from build123d import *

# Parameters (mm, degrees)
F0_W     = 18.4755190939
F0_H     = 19.05
F1_DEPTH = 12.7
F2_DEPTH = 76.2
F4_DEPTH = 12.7
F3_W     = 19.05
F3_H     = 19.05
F5_DEPTH = 25.4


# Not quite as in the source:
# - a feature names something its author has since deleted; it is built from what else it names


with BuildPart() as f1:
    # F0 (on Top) → F1 (new body)
    with BuildSketch(Plane.XY):
        with BuildLine():
            Line((34.1462217655, 9.525), (-48.9782591407, 9.525))
            ThreePointArc((-48.9782591407, 9.525), (-58.5032591407, 0), (-48.9782591407, -9.525))
            Line((-48.9782591407, -9.525), (34.1462217655, -9.525))
            Line((34.1462217655, -9.525), (34.1462217655, 9.525))
        make_face()
        with Locations((43.3839813124, 0)):
            Rectangle(F0_W, F0_H)
    extrude(amount=F1_DEPTH)

    # F0 (on Top) → F2 (join)
    with BuildSketch(Plane.XY):
        with Locations((43.3839813124, 0)):
            Rectangle(F0_W, F0_H)
    extrude(amount=F2_DEPTH)

    # F3 (on face) → F4 (join)
    with BuildSketch(Plane.XY.offset(76.2)):
        Polygon((52.6217408593, -9.525), (34.1462217655, -9.525), (34.1462217655, -219.075), (53.1962217655, -219.075), (53.1962217655, -9.525), align=None)
    extrude(amount=-F4_DEPTH)

    # F3 (on face) → F5 (join)
    with BuildSketch(Plane.XY.offset(76.2)):
        with Locations((43.6712217655, -228.6)):
            Rectangle(F3_W, F3_H)
    extrude(amount=-F5_DEPTH)


with BuildPart() as f6_1:
    # F6: copy of F1
    add(f1.part)


solid = f1.part
Read the model definition and answer for the solid it produces. Units are mm, in the model's axes. A direction names the side the tool comes from. Give positions to 0.01 mm unless a question says otherwise; leave off trailing zeros. Loops run counter-clockwise (first coordinate to the right, second up) from the corner with the lowest first, then second, coordinate; pieces in that order, holes last. Notation, with made-up numbers: (88.25, 9) - (128.25, 9) arc R25 cw to (128.25, 21) - close; hole circle Ø11 at (81, 41.25). An arc over 180 degrees is marked (long way). Answer as CSV lines item,"result". Start each with the question number.
1) Determine the mould class of faces 1 (the face through (44, -113, 76.2)), 2 (the face through (44, -219.075, 57)), 3 (the face through (25, 9.525, 12)) for opening direction Y: released by +Y, released by -Y, zero draft, split by the parting line, or undercut.
2) Each of these flat-tipped pins is pushed along its axis until it touches: pin 1 Ø0.6 at (x, z) = (53, 72) entering from +Y (3 decimals); pin 2 Ø15 at (y, z) = (1, 24.5) entering from +X; pin 3 Ø21 at (x, y) = (41, -80) entering from -Z. Where does it stop, or does it pass through?
3) Straight lines are drawn through the part: L1, parallel to Z at x = 43, y = -100; L2, parallel to X at y = -29.5, z = 64.5; L3, parallel to Y at x = 40, z = 12.5 (3 decimals). For each, find the intervals that lie inside material, in ascending order. Write a range as from..to.
4) Find section A-A (x = 38). Write down the section's boundary in (y, z) (3 decimals).
5) Find section D-D (x = 23). Write down the section's boundary in (y, z) (3 decimals), then the cut area to 3 significant figures.
6) Which of the six approach directions +Z, -Z, +X, -X, +Y, -Y give full straight-line access (tool end or side, diameter ignored) to faces 4 (the face through (24, -9.525, 10)), 5 (the face through (44, -228, 50.8)), 6 (the face through (-13, 0, 12.7))?
7) Find section C-C (y = 0). Write down the section's boundary in (x, z).
8) Find section B-B (z = 20). Write down the section's boundary in (x, y) (3 decimals).
Findings below:
1,face 1,"zero draft"
1,face 2,"undercut"
1,face 3,"released by +Y"
2,pin 1,"y = -9.525"
2,pin 2,"x = 52.62"
2,pin 3,"z = 63.5"
3,L1,"63.5..76.2"
3,L2,"34.15..53.2"
3,L3,"-9.525..9.525"
4,outline,"(-238.125, 50.8) - (-219.075, 50.8) - (-219.075, 63.5) - (-9.525, 63.5) - (-9.525, 0) - (9.525, 0) - (9.525, 76.2) - (-238.125, 76.2) - close"
5,outline,"(-9.525, 0) - (9.525, 0) - (9.525, 12.7) - (-9.525, 12.7) - close"
5,area,"242 mm^2"
6,face 4,"-Z, +X, -X"
6,face 5,"-Z, +X, -X, -Y"
6,face 6,"+Z, -X, +Y, -Y"
7,outline,"(-58.5, 0) - (52.62, 0) - (52.62, 76.2) - (34.15, 76.2) - (34.15, 12.7) - (-58.5, 12.7) - close"
8,outline,"(34.146, -9.525) - (52.622, -9.525) - (52.622, 9.525) - (34.146, 9.525) - close"
